```python
from build123d import *

# Parameters (mm, degrees)
SKETCH_1_R          = 5
EXTRUDE_1_DEPTH     = 68
SKETCH_2_W          = 68.768815545
SKETCH_2_H          = 54
CUT_EXTRUDE_1_DEPTH = 106.470374987
SKETCH_3_R          = 5
SKETCH_3_R_2        = 2.5
CUT_EXTRUDE_2_DEPTH = 106.470374987
SKETCH_4_R          = 1.5
CUT_EXTRUDE_3_DEPTH = 106.470374987


with BuildPart() as part:
    # ｽｹｯﾁ1 → ﾎﾞｽ - 押し出し1 (new body)
    with BuildSketch(Plane.XY):
        with BuildLine():
            Line((0, 0), (0, -40))
            Line((0, -40), (-50, -40))
            ThreePointArc((-50, -40), (-70, -20), (-50, 0))
            Line((-50, 0), (0, 0))
        make_face()
        with Locations((-50, -20)):
            Circle(SKETCH_1_R, mode=Mode.SUBTRACT)
    extrude(amount=EXTRUDE_1_DEPTH)

    # ｽｹｯﾁ2 → ｶｯﾄ - 押し出し1 (cut, through all)
    with BuildSketch(Plane(origin=(0, 0, 0), x_dir=(1, 0, 0), z_dir=(0, 1, 0))):
        with Locations((-41.384407773, -34)):
            Rectangle(SKETCH_2_W, SKETCH_2_H)
    extrude(amount=-CUT_EXTRUDE_1_DEPTH, mode=Mode.SUBTRACT)

    # ｽｹｯﾁ3 → ｶｯﾄ - 押し出し2 (cut, through all)
    with BuildSketch(Plane(origin=(0, 0, 0), x_dir=(0, 0, -1), z_dir=(1, 0, 0))):
        with Locations(Location((-34, -20, 0), (0, 0, 90))):
            Circle(SKETCH_3_R)
        with Locations(Location((-54, -20, 0), (0, 0, 90))):
            Circle(SKETCH_3_R_2)
        with Locations((-14, -20)):
            Circle(SKETCH_3_R_2)
    extrude(amount=-CUT_EXTRUDE_2_DEPTH, mode=Mode.SUBTRACT)

    # ｽｹｯﾁ4 → ｶｯﾄ - 押し出し3 (cut, through all)
    with BuildSketch(Plane(origin=(0, 0, 0), x_dir=(-1, 0, 0), z_dir=(0, 0, -1))):
        with Locations((12, -10)):
            Circle(SKETCH_4_R)
        with Locations(Location((12, -30, 0), (0, 0, 180))):
            Circle(SKETCH_4_R)
    extrude(amount=-CUT_EXTRUDE_3_DEPTH, mode=Mode.SUBTRACT)


solid = part.part
```
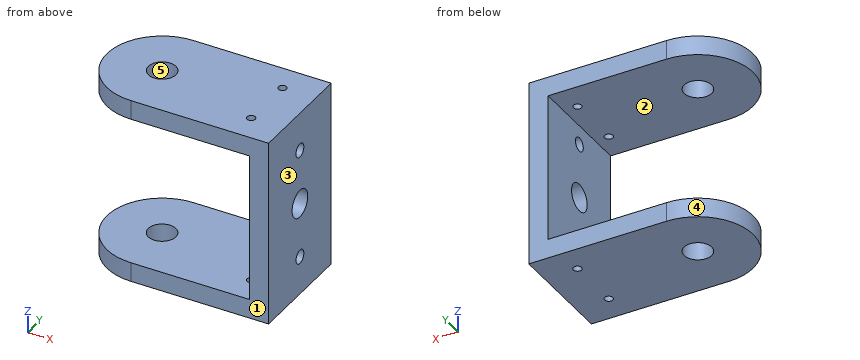
Part model, mm, in its own coordinate system. Face numbers are marked on the shaded views. A direction names the side the tool comes from. Coordinates: 2 decimals unless noted, no trailing zeros. Write each loop counter-clockwise with the first axis right and the second up, starting at its lowest first coordinate (ties: lowest second). Pieces come first, ordered by that corner, then holes.
Item 1: Slice it at B-B (y = -20). Write the cut outline in (x, z), and give its area (3 significant figures).
Item 2: Which spindle directions (+Z, -Z, +X, -X, +Y, -Y) get a long thin tool onto all of the face, cutting with end or side? Do the marked faces 1 and 2. Say none if no direction does.
Item 3: Pin check, flat tips, straight feed: pin 1 (6 mm diameter, centred on x = -50, y = -20, fed in from +Z); pin 2 (4 mm diameter, centred on y = -32.5, z = 21, fed in from -X). Stop position of each tip, or through.
Item 4: Slice it at A-A (x = -12). Write the cut outline in (y, z), and give its area (3 significant figures).
Item 5: Probe line 1 (Y direction, x = -12, z = 2.5); line 2 (Z direction, x = -53, y = -10); line 3 (Y direction, x = -50, z = 65). List the from-to ranges inside material, lowest first.
Item 6: Slice it at C-C (z = 34). Write the cut outline in (x, y), and give its area (3 significant figures).
Item 7: Slice it at D-D (y = -10). Write the cut outline in (x, z).
Item 8: Mould opens along X. For the marked faces 3, 4 and 5 say: released by +X, released by -X, zero draft, split by the parting line, or undercut.
Results found:
1. outline: (-70, 0) - (-55, 0) - (-55, 7) - (-70, 7) - close; (-70, 61) - (-55, 61) - (-55, 68) - (-70, 68) - close; (-45, 0) - (0, 0) - (0, 11.5) - (-7, 11.5) - (-7, 7) - (-45, 7) - close; (-45, 61) - (-7, 61) - (-7, 56.5) - (0, 56.5) - (0, 68) - (-45, 68) - close; (-7, 16.5) - (0, 16.5) - (0, 29) - (-7, 29) - close; (-7, 39) - (0, 39) - (0, 51.5) - (-7, 51.5) - close
1. area: 1,080 mm2
2. face 1: +Z, -Z, +X, -X, -Y
2. face 2: -X, +Y, -Y
3. pin 1: passes through
3. pin 2: stops at x = -7
4. outline: (-40, 0) - (-31.5, 0) - (-31.5, 7) - (-40, 7) - close; (-40, 61) - (-31.5, 61) - (-31.5, 68) - (-40, 68) - close; (-28.5, 0) - (-11.5, 0) - (-11.5, 7) - (-28.5, 7) - close; (-28.5, 61) - (-11.5, 61) - (-11.5, 68) - (-28.5, 68) - close; (-8.5, 0) - (0, 0) - (0, 7) - (-8.5, 7) - close; (-8.5, 61) - (0, 61) - (0, 68) - (-8.5, 68) - close
4. area: 476 mm2
5. line 1: y = -40 to -31.5, -28.5 to -11.5, -8.5 to 0
5. line 2: z = 0 to 7, 61 to 68
5. line 3: y = -40 to -25, -15 to 0
6. outline: (-7, -40) - (0, -40) - (0, -25) - (-7, -25) - close; (-7, -15) - (0, -15) - (0, 0) - (-7, 0) - close
6. area: 210 mm2
7. outline: (-67.32, 0) - (-13.5, 0) - (-13.5, 7) - (-67.32, 7) - close; (-67.32, 61) - (-13.5, 61) - (-13.5, 68) - (-67.32, 68) - close; (-10.5, 0) - (0, 0) - (0, 68) - (-10.5, 68) - (-10.5, 61) - (-7, 61) - (-7, 7) - (-10.5, 7) - close
8. face 3: released by +X
8. face 4: released by -X
8. face 5: undercut
